Work out the finished part from the listing and answer in its coordinate system (mm). A direction names the side the tool comes from. Round coordinates to 2 decimals unless told otherwise and drop trailing zeros. Order: outer loops, then holes, each group sorted by start corner. A loop starts at its lowest first (then second) coordinate and runs counter-clockwise, first axis right, second up. Notation, with made-up numbers: M 35,-31.5 L 60,-31.5 A5 ccw 60,-26.5 Z; hole C 87.5,31.25 d9. An arc over 180 degrees is marked long. Return JSON: item names as keys, results as strings.
from build123d import *

# Parameters (mm, degrees)
BOSS_EXTRUDE1_DEPTH = 5
SKETCH2_R           = 1.3
CUT_EXTRUDE1_DEPTH  = 14.35984761
SKETCH3_R           = 1.3
CUT_EXTRUDE2_DEPTH  = 14.591735948
FILLET1_R           = 1
FILLET2_R           = 1


with BuildPart() as part:
    # Sketch1 → Boss-Extrude1 (new body)
    with BuildSketch(Plane(origin=(0, 0, 0), x_dir=(1, 0, 0), z_dir=(0, 1, 0))):
        with BuildLine():
            Line((2.3, -6.88444102), (2.3, -1.766352173))
            ThreePointArc((2.3, -1.766352173), (2.745906044, -0.932737905), (2.9, 0))
            Line((2.9, 0), (8, 0))
            Line((8, 0), (8, 2.9))
            Line((8, 2.9), (0, 2.9))
            ThreePointArc((0, 2.9), (-2.601194082, 1.282103486), (-2.3, -1.766352173))
            Line((-2.3, -1.766352173), (-2.3, -6.88444102))
            Line((-2.3, -6.88444102), (-0.3, -6.88444102))
            Line((-0.3, -6.88444102), (-0.3, -2.88444102))
            Line((-0.3, -2.88444102), (-0.3, -1.469693846))
            ThreePointArc((-0.3, -1.469693846), (0, 1.5), (0.3, -1.469693846))
            Line((0.3, -1.469693846), (0.3, -2.88444102))
            Line((0.3, -2.88444102), (0.3, -6.88444102))
            Line((0.3, -6.88444102), (2.3, -6.88444102))
        make_face()
    extrude(amount=BOSS_EXTRUDE1_DEPTH)

    # Sketch2 → Cut-Extrude1 (cut, through all)
    with BuildSketch(Plane.ZY.offset(2.3)):
        with Locations((4.325396597, 2.5)):
            Circle(SKETCH2_R)
    extrude(amount=-CUT_EXTRUDE1_DEPTH, mode=Mode.SUBTRACT)

    # Sketch3 → Cut-Extrude2 (cut, through all)
    with BuildSketch(Plane(origin=(0, 0, -2.9), x_dir=(-1, 0, 0), z_dir=(0, 0, -1))):
        with Locations((-5.5, 2.5)):
            Circle(SKETCH3_R)
    extrude(amount=-CUT_EXTRUDE2_DEPTH, mode=Mode.SUBTRACT)

    # Fillet1
    fillet1_edges = [part.edges().sort_by_distance(p)[0] for p in [
        (1.3, 0, 6.88444102),
        (-1.3, 0, 6.88444102),
        (-1.3, 5, 6.88444102),
        (1.3, 5, 6.88444102),
    ]]
    fillet(fillet1_edges, radius=FILLET1_R)

    # Fillet2
    fillet2_edges = [part.edges().sort_by_distance(p)[0] for p in [
        (8, 0, -1.45),
        (8, 5, -1.45),
    ]]
    fillet(fillet2_edges, radius=FILLET2_R)


solid = part.part
Item 1: Which of the six approach directions +Z, -Z, +X, -X, +Y, -Y give full straight-line access (tool end or side, diameter ignored) to faces 5 (the flat face through (-2.3, 4, 3)), 6 (the flat face through (2.3, 1, 3)), 7 (the flat face through (0.3, 4, 4))?
Output:
{"face 5": "+Z, -X, +Y, -Y", "face 6": "+Z, +X, +Y, -Y", "face 7": "+Z, +Y, -Y"}
Item 2: Find section A-A (z = -2). Determine the outline of the cut face in (x, y), plus the area to 3 significant figures.
Output:
{"outline": "M -2.1,0 L 7,0 A1 ccw 8,1 L 8,4 A1 ccw 7,5 L -2.1,5 Z; hole C 5.5,2.5 d2.6", "area": "44.8 mm^2"}
Item 3: Find section B-B (x = 5.5). Determine the outline of the cut face in (y, z), plus the area to 3 significant figures.
Output:
{"outline": "M 0,-2.9 L 1.2,-2.9 L 1.2,0 L 0,0 Z; M 3.8,-2.9 L 5,-2.9 L 5,0 L 3.8,0 Z", "area": "6.96 mm^2"}
Item 4: Find section C-C (y = 2.5). Determine the outline of the cut face in (x, z), plus the area to 3 significant figures.
Output:
{"outline": "M -2.3,1.77 A2.9 ccw 0,-2.9 L 4.2,-2.9 L 4.2,0 L 2.9,0 A2.9 ccw 2.3,1.77 L 2.3,3.03 L 0.3,3.03 L 0.3,1.47 A1.5 cw long -0.3,1.47 L -0.3,3.03 L -2.3,3.03 Z; M -2.3,5.63 L -0.3,5.63 L -0.3,6.88 L -2.3,6.88 Z; M 0.3,5.63 L 2.3,5.63 L 2.3,6.88 L 0.3,6.88 Z; M 6.8,-2.9 L 8,-2.9 L 8,0 L 6.8,0 Z", "area": "34.7 mm^2"}
Item 5: Consider line 1 along Y through (x, z) = (2.25, 4.25); line 2 along X through (y, z) = (3.9, 4.75); line 3 along Z through (x, y) = (3, 2.1). Determine where each line is inside the solid, lowest interval first. Write a range as [from, to].
Output:
{"line 1": "y = [0, 1.2], [3.8, 5]", "line 2": "x = [-2.3, -0.3], [0.3, 2.3]", "line 3": "z = [-2.9, 0]"}
Item 6: Each of these flat-tipped pins is pushed along its axis until it touches: pin 1 (2.5 mm diameter, centred on y = 2.5, z = 4.33, fed in from -X); pin 2 (1.5 mm diameter, centred on y = 1.5, z = 4, fed in from -X). Where does it stop, or does it pass through?
Output:
{"pin 1": "passes through", "pin 2": "stops at x = -2.3"}
Item 7: Find section D-D (z = 2.5). Determine the outline of the cut face in (x, y).
Output:
{"outline": "M -2.3,0 L -0.3,0 L -0.3,5 L -2.3,5 Z; M 0.3,0 L 2.3,0 L 2.3,5 L 0.3,5 Z"}
Item 8: The mould has two halves that part along Z. Classify faces 1 (the cylindrical face through (1.286, 2.557, 3.027)), 2 (the cylindrical face through (-0.06, 2.46, -1.5)), 3 (the flat face through (2, 0, 0)), 4 (the cylindrical face through (-1.3, 4.7, 6.6)): pulls with the +Z half, pulls with the -Z half, needs draft (parallel to the pull), parting line crosses it, or undercut.
Output:
{"face 1": "undercut", "face 2": "undercut", "face 3": "needs draft", "face 4": "pulls with the +Z half"}
